from build123d import *

# Parameters (mm, degrees)
SKETCH1_R           = 2
SKETCH1_R_2         = 1.5
SKETCH1_W           = 30
SKETCH1_H           = 3
SKETCH1_W_2         = 3
SKETCH1_H_2         = 30
SKETCH1_W_3         = 5
SKETCH1_H_3         = 19.9734
SKETCH1_H_4         = 19.45
BOSS_EXTRUDE1_DEPTH = 3


with BuildPart() as part:
    # Sketch1 → Boss-Extrude1 (new body)
    with BuildSketch(Plane(origin=(-12.611770594, -16.696126479, 0), x_dir=(0, -1, 0), z_dir=(0, 0, 1))):
        Polygon((-213.696126479, 12.611770594), (-213.696126479, 392.611770594), (-16.696126479, 392.611770594), (-16.696126479, 342.611770594), (-44.166313492, 283.701764437), (-52.593278212, 202.611770594), (-44.166313492, 121.521776752), (-16.696126479, 62.611770594), (-16.696126479, 12.611770594), align=None)
        with Locations((-207.593278212, 103.411770594)):
            Circle(SKETCH1_R, mode=Mode.SUBTRACT)
        with Locations((-69.593278212, 103.411770594)):
            Circle(SKETCH1_R, mode=Mode.SUBTRACT)
        with Locations((-93.593278212, 29.411770594)):
            Circle(SKETCH1_R, mode=Mode.SUBTRACT)
        with Locations((-207.593278212, 39.411770594)):
            Circle(SKETCH1_R, mode=Mode.SUBTRACT)
        with Locations((-200.179850585, 21.491770594)):
            Circle(SKETCH1_R_2, mode=Mode.SUBTRACT)
        with Locations((-58.093278212, 311.89748488)):
            Circle(SKETCH1_R_2, mode=Mode.SUBTRACT)
        with Locations((-200.196126479, 383.111770594)):
            Circle(SKETCH1_R_2, mode=Mode.SUBTRACT)
        with Locations((-71.696126479, 383.111770594)):
            Circle(SKETCH1_R_2, mode=Mode.SUBTRACT)
        with Locations((-58.093278212, 93.326056309)):
            Circle(SKETCH1_R_2, mode=Mode.SUBTRACT)
        with Locations((-71.679850585, 21.491770594)):
            Circle(SKETCH1_R_2, mode=Mode.SUBTRACT)
        Polygon((-209.593278212, 95.411770594), (-195.593278212, 109.411770594), (-81.593278212, 109.411770594), (-63.593278212, 91.411770594), (-63.593278212, 35.411770594), (-97.593278212, 35.411770594), (-109.018462266, 27.411770594), (-201.593276784, 27.411770594), (-201.593276784, 47.411770594), (-209.593278212, 47.411770594), align=None, mode=Mode.SUBTRACT)
        with Locations((-171.679850585, 21.491770594)):
            Rectangle(SKETCH1_W, SKETCH1_H, mode=Mode.SUBTRACT)
        with Locations((-101.679850585, 21.491770594)):
            Rectangle(SKETCH1_W, SKETCH1_H, mode=Mode.SUBTRACT)
        with Locations((-58.093278212, 56.89748488)):
            Rectangle(SKETCH1_W_2, SKETCH1_H_2, mode=Mode.SUBTRACT)
        with Locations((-58.093278212, 129.754627737)):
            Rectangle(SKETCH1_W_2, SKETCH1_H_2, mode=Mode.SUBTRACT)
        with Locations((-58.093278212, 202.611770594)):
            Rectangle(SKETCH1_W_2, SKETCH1_H_2, mode=Mode.SUBTRACT)
        with Locations((-58.093278212, 275.468913452)):
            Rectangle(SKETCH1_W_2, SKETCH1_H_2, mode=Mode.SUBTRACT)
        with Locations((-58.093278212, 348.326056309)):
            Rectangle(SKETCH1_W_2, SKETCH1_H_2, mode=Mode.SUBTRACT)
        with Locations((-101.696126479, 383.111770594)):
            Rectangle(SKETCH1_W, SKETCH1_H, mode=Mode.SUBTRACT)
        with Locations((-171.696126479, 383.111770594)):
            Rectangle(SKETCH1_W, SKETCH1_H, mode=Mode.SUBTRACT)
        Polygon((-69.353278212, 118.571770594), (-113.803278212, 118.571770594), (-113.803278212, 277.321770594), (-174.353278212, 277.321770594), (-174.353278212, 360.595170594), (-69.353278212, 360.595170594), align=None, mode=Mode.SUBTRACT)
        with Locations((-182.923278212, 287.308470594)):
            Rectangle(SKETCH1_W_3, SKETCH1_H_3, mode=Mode.SUBTRACT)
        with Locations((-182.923278212, 307.890170594)):
            Rectangle(SKETCH1_W_3, SKETCH1_H_4, mode=Mode.SUBTRACT)
        with Locations((-182.923278212, 328.210170594)):
            Rectangle(SKETCH1_W_3, SKETCH1_H_4, mode=Mode.SUBTRACT)
        with Locations((-182.923278212, 348.530170594)):
            Rectangle(SKETCH1_W_3, SKETCH1_H_4, mode=Mode.SUBTRACT)
    extrude(amount=BOSS_EXTRUDE1_DEPTH)


solid = part.part
The model under review builds one solid part; all positions refer to its coordinate system, in mm. A direction names the side the tool comes from. Coordinates: 2 decimals unless noted, no trailing zeros. Loops run counter-clockwise (first coordinate to the right, second up) from the corner with the lowest first, then second, coordinate; pieces in that order, holes last.
(1) Tool access review of faces 1 (the flat face through (89.702, 185.995, 1.479)), 2 (the flat face through (231.113, 31.625, 1.479)), 3 (the flat face through (235, 119, 0)): name each direction out of +Z, -Z, +X, -X, +Y, -Y from which nothing blocks a thin tool from reaching the whole face with its end or side.
Determined:
face 1: +Z, -Z
face 2: +Z, -Z, -Y
face 3: -Z, +X, -X, +Y, -Y
(2) Wall thickness on L1, parallel to X at y = 120, z = 1.65; L2, parallel to X at y = 147, z = 0.7; L3, parallel to X at y = 162.5, z = 1.1: over which ranges is each line inside the solid? List them lowest first.
Determined:
L1: x = 0 to 14.8, 96.8 to 264.71, 347.98 to 380
L2: x = 0 to 7.38, 10.38 to 14.8, 96.8 to 264.71, 347.98 to 369, 372 to 380
L3: x = 0 to 7.38, 10.38 to 14.8, 96.8 to 369, 372 to 380
(3) Consider section C-C, the plane z = 1.3. Give the number of separate pieces and of enclosed holes in the cut face, plus the area to 3 significant figures.
Determined:
separate pieces: 1
enclosed holes: 25
area: 39,800 mm2
(4) Consider section B-B, the plane x = 229.5. Give the boundary of the cut face in (y, z).
Determined:
outline: (31.79, 0) - (52.66, 0) - (52.66, 3) - (31.79, 3) - close; (97.11, 0) - (197, 0) - (197, 3) - (97.11, 3) - close
(5) Draft analysis for pull direction Y (two halves, no side actions). For faces 4 (the flat face through (87.926, 56.023, 1.479)), 5 (the flat face through (235, 119, 3)), 6 (the flat face through (150.023, 31.743, 1.479)), 7 (the flat face through (18.856, 86.53, 1.479)), state which applies: +Y half, -Y half, draft (parallel to the pull), parting line (faces both ways), or undercut.
Determined:
face 4: undercut
face 5: draft
face 6: -Y half
face 7: undercut
(6) Consider section A-A, the plane x = 289.5. Give the boundary of the cut face in (y, z).
Determined:
outline: (18.89, 0) - (52.66, 0) - (52.66, 3) - (18.89, 3) - close; (157.66, 0) - (163.73, 0) - (163.73, 3) - (157.66, 3) - close; (168.73, 0) - (197, 0) - (197, 3) - (168.73, 3) - close
(7) Insertion check: P1, Ø8, axis at x = 178, y = 57, coming from the +Z side; P2, Ø1.5, axis at x = 272, z = 2, coming from the -Y side; P3, Ø0.9, axis at x = 190.5, z = 1.5, coming from the -Y side. Each pin has a flat end and moves straight along its axis. Give the tip position at first contact, or say it passes through.
Determined:
P1: passes through
P2: stops at y = 26.7
P3: stops at y = 35.8
(8) Consider section D-D, the plane x = 154.5. Give the boundary of the cut face in (y, z), plus the area to 3 significant figures.
Determined:
outline: (32.21, 0) - (52.66, 0) - (52.66, 3) - (32.21, 3) - close; (97.11, 0) - (197, 0) - (197, 3) - (97.11, 3) - close
area: 361 mm2
